CAD build for the part. Positions are in the model's coordinates, mm. A direction names the side the tool comes from. Round coordinates to 2 decimals unless told otherwise and drop trailing zeros. Loops run counter-clockwise (first coordinate to the right, second up) from the corner with the lowest first, then second, coordinate; pieces in that order, holes last. Notation, with made-up numbers: (48, 86) - (94, 86) arc R19 cw to (94, 91) - close; hole circle Ø6 at (-10.75, 10.25). An arc over 180 degrees is marked (long way). Use one line per item in the form item = value.
from build123d import *

# Parameters (mm, degrees)
F1_DEPTH = 35
F3_DEPTH = 2
F4_R     = 2.5
F5_DEPTH = 25
F6_W     = 8.2
F6_H     = 3.2
F7_DEPTH = 7
F8_W     = 30
F8_H     = 18.9
F9_DEPTH = 5


with BuildPart() as f1:
    # F0 (on Front) → F1 (new body)
    with BuildSketch(Plane.XZ):
        Polygon((-15, 11.5), (-32.5, 11.5), (-32.5, -11.5), (-25, -11.5), (-25, -8.5), (-29.5, -8.5), (-29.5, 3.5), (-30.5, 3.5), (-30.5, 8.5), (-29.5, 8.5), (29.5, 8.5), (29.5, -8.5), (25, -8.5), (25, -11.5), (32.5, -11.5), (32.5, 11.5), (15, 11.5), (15, 19.5), (0, 19.5), (-15, 19.5), align=None)
    extrude(amount=F1_DEPTH)

    # F2 (on face) → F3 (join)
    with BuildSketch(Plane(origin=(0, 0, 0), x_dir=(-1, 0, 0), z_dir=(0, 1, 0))):
        Polygon((-15, 11.5), (-32.5, 11.5), (-32.5, -11.5), (-25, -11.5), (25, -11.5), (32.5, -11.5), (32.5, 11.5), (15, 11.5), (15, 19.5), (-15, 19.5), align=None)
    extrude(amount=-F3_DEPTH)

    # F4 (on face) → F5 (cut)
    with BuildSketch(Plane.XY.offset(19.5)):
        with Locations((0, -8.5)):
            Circle(F4_R)
    extrude(amount=-F5_DEPTH, mode=Mode.SUBTRACT)

    # F6 (on face) → F7 (cut)
    with BuildSketch(Plane.XY.offset(19.5)):
        with Locations((-8.2, -8.5)):
            Rectangle(F6_W, F6_H)
        with Locations((8.2, -8.5)):
            Rectangle(F6_W, F6_H)
    extrude(amount=-F7_DEPTH, mode=Mode.SUBTRACT)

    # F8 (on face) → F9 (cut)
    with BuildSketch(Plane.XY.offset(19.5)):
        with Locations((0, -25.55)):
            Rectangle(F8_W, F8_H)
    extrude(amount=-F9_DEPTH, mode=Mode.SUBTRACT)


solid = f1.part
1) Slice it at C-C (z = 16.5). Write the cut outline in (x, y), plus the area to 3 significant figures.
Report:
outline = (-15, -16.1) - (15, -16.1) - (15, 0) - (-15, 0) - close; hole (-12.3, -10.1) - (-4.1, -10.1) - (-4.1, -6.9) - (-12.3, -6.9) - close; hole circle Ø5 at (0, -8.5); hole (4.1, -10.1) - (12.3, -10.1) - (12.3, -6.9) - (4.1, -6.9) - close
area = 411 mm^2
2) Two-plate mould, pull along Z, no slides. Class faces 1 (the flat face through (32.5, -17, 0)), 2 (the flat face through (-30.5, -18, 6)), 3 (the flat face through (-24, -17, 11.5)): +Z half, -Z half, draft (parallel to the pull), parting line (faces both ways), or undercut.
Report:
face_1 = draft
face_2 = undercut
face_3 = +Z half
3) Drill centre lines: probe 1 along Y at (x, z) = (0, 16.5); probe 2 along Y at (x, z) = (0, 14); probe 3 along X at (y, z) = (-8, 16). Where is each one in solid material? Low to high.
Report:
probe_1 = -16.1 to -11, -6 to 0
probe_2 = -35 to -11, -6 to 0
probe_3 = -15 to -12.3, -4.1 to -2.45, 2.45 to 4.1, 12.3 to 15
4) Tool access for faces 4 (the flat face through (0, -25, 14.5)), 5 (the flat face through (8, -8, 12.5)), 6 (the flat face through (-27, -18, -8.5)), 7 (the flat face through (-15, -13, 15)): list every direction of +Z, -Z, +X, -X, +Y, -Y with a clear straight run to the whole face (end or side of a thin tool).
Report:
face_4 = +Z, +X, -X, -Y
face_5 = +Z
face_6 = -Y
face_7 = +Z, -X, +Y, -Y
5) Flat gauge pins, fed straight in: pin 1 (2 mm diameter, centred on x = 16, z = -0.5, fed in from -Y); pin 2 (1.5 mm diameter, centred on x = 24, y = -16, fed in from +Z); pin 3 (10 mm diameter, centred on x = 4.5, y = -26, fed in from +Z). Where does each tip first touch, or does it go through?
Report:
pin_1 = -2
pin_2 = 11.5
pin_3 = 14.5
6) Slice it at D-D (y = -12). Write the cut outline in (x, z).
Report:
outline = (-32.5, -11.5) - (-25, -11.5) - (-25, -8.5) - (-29.5, -8.5) - (-29.5, 3.5) - (-30.5, 3.5) - (-30.5, 8.5) - (29.5, 8.5) - (29.5, -8.5) - (25, -8.5) - (25, -11.5) - (32.5, -11.5) - (32.5, 11.5) - (15, 11.5) - (15, 19.5) - (-15, 19.5) - (-15, 11.5) - (-32.5, 11.5) - close
7) Slice it at B-B (x = -1.5). Write the cut outline in (y, z), plus the area to 4 significant figures.
Report:
outline = (-35, 8.5) - (-10.5, 8.5) - (-10.5, 19.5) - (-16.1, 19.5) - (-16.1, 14.5) - (-35, 14.5) - close; (-6.5, 8.5) - (-2, 8.5) - (-2, -11.5) - (0, -11.5) - (0, 19.5) - (-6.5, 19.5) - close
area = 286.5 mm^2
